```python
from build123d import *

# Parameters (mm, degrees)
SKETCH_1_R          = 18
LASHENA_DEPTH       = 30
CUT_EXTRUDEA_DEPTH  = 30
WWW_KYTOOL_CN_COUNT = 16
SKETCH_3_W          = 35.542909486
SKETCH_3_H          = 27
CUT_EXTRUDE_2_DEPTH = 30
SKETCH_4_R          = 1.5
CUT_EXTRUDE_3_DEPTH = 60
SKETCH_5_R          = 1.5
EXTRUDE_3_DEPTH     = 3
CUT_EXTRUDE_5_DEPTH = 3


with BuildPart() as part:
    # 草图1 → LaShenA (new body)
    with BuildSketch(Plane.XY):
        Circle(SKETCH_1_R)
    extrude(amount=LASHENA_DEPTH)

    # SketchA → Cut-ExtrudeA (cut)
    with BuildSketch(Plane.XY.offset(30)):
        with BuildLine():
            ThreePointArc((0.423212707, 13.493364703), (0, 13.5), (-0.423212707, 13.493364703))
            ThreePointArc((-0.423212707, 13.493364703), (-0.952770902, 13.685686791), (-1.20440395, 14.18977059))
            add(Edge.make_bspline(
                [(-1.20440395, 14.18977059), (-1.226562505, 14.455224305), (-1.213843633, 14.773889884), (-1.273675597, 15.110607864), (-1.299119688, 15.21139578), (-1.321432077, 15.29109757), (-1.349914152, 15.382250837), (-1.385146673, 15.484587535), (-1.427834192, 15.597770763), (-1.478623281, 15.721446817), (-1.538159915, 15.855229004), (-1.607069773, 15.998703507), (-1.685962928, 16.151428337), (-1.775430978, 16.312934487), (-1.876046532, 16.482726463), (-1.98836201, 16.660283053), (-2.112908684, 16.845058076), (-2.250195688, 17.036481179), (-2.400709063, 17.233958676), (-2.56491084, 17.43687441), (-2.743238138, 17.644590662), (-2.936102365, 17.856449073), (-3.14388814, 18.07177164), (-3.447378451, 18.368492697), (-3.689495989, 18.585006365), (-3.858042439, 18.727457792)],
                knots=[0.122308221, 0.122308221, 0.122308221, 0.122308221, 0.250610689, 0.276296194, 0.287604067, 0.300967916, 0.316387742, 0.333863545, 0.353395324, 0.37498308, 0.398626813, 0.424326522, 0.452082207, 0.48189387, 0.513761509, 0.547685125, 0.583664717, 0.621700286, 0.661791832, 0.703939355, 0.748142854, 0.79440233, 0.842717782, 0.893089212, 1, 1, 1, 1], degree=3))
            ThreePointArc((-3.858042439, 18.727457792), (0, 19.120726106), (3.858042439, 18.727457792))
            add(Edge.make_bspline(
                [(1.20440395, 14.18977059), (1.226562505, 14.455224305), (1.213843633, 14.773889884), (1.273675597, 15.110607864), (1.299119688, 15.21139578), (1.321432077, 15.29109757), (1.349914152, 15.382250837), (1.385146673, 15.484587535), (1.427834192, 15.597770763), (1.478623281, 15.721446817), (1.538159915, 15.855229004), (1.607069773, 15.998703507), (1.685962928, 16.151428337), (1.775430978, 16.312934487), (1.876046532, 16.482726463), (1.98836201, 16.660283053), (2.112908684, 16.845058076), (2.250195688, 17.036481179), (2.400709063, 17.233958676), (2.56491084, 17.43687441), (2.743238138, 17.644590662), (2.936102365, 17.856449073), (3.14388814, 18.07177164), (3.447378451, 18.368492697), (3.689495989, 18.585006365), (3.858042439, 18.727457792)],
                knots=[0.122308221, 0.122308221, 0.122308221, 0.122308221, 0.250610689, 0.276296194, 0.287604067, 0.300967916, 0.316387742, 0.333863545, 0.353395324, 0.37498308, 0.398626813, 0.424326522, 0.452082207, 0.48189387, 0.513761509, 0.547685125, 0.583664717, 0.621700286, 0.661791832, 0.703939355, 0.748142854, 0.79440233, 0.842717782, 0.893089212, 1, 1, 1, 1], degree=3))
            ThreePointArc((1.20440395, 14.18977059), (0.952770902, 13.685686791), (0.423212707, 13.493364703))
        make_face()
    cut_extrudea = extrude(amount=-CUT_EXTRUDEA_DEPTH, mode=Mode.SUBTRACT)

    # www.KYTool.cn: Cut-ExtrudeA ×16 about axis
    www_kytool_cn_axis = Axis((0, 0, -80.9), (0, 0, 1))
    for i in range(1, WWW_KYTOOL_CN_COUNT):
        add(cut_extrudea.rotate(www_kytool_cn_axis, i * 360 / WWW_KYTOOL_CN_COUNT), mode=Mode.SUBTRACT)

    # 草图3 → 切除-拉伸2 (cut, symmetric)
    with BuildSketch(Plane(origin=(0, 0, 0), x_dir=(1, 0, 0), z_dir=(0, 1, 0))):
        with Locations((0, -13.5)):
            Rectangle(SKETCH_3_W, SKETCH_3_H)
    extrude(amount=CUT_EXTRUDE_2_DEPTH, both=True, mode=Mode.SUBTRACT)

    # 草图4 → 切除-拉伸3 (cut)
    with BuildSketch(Plane.XY.offset(30)):
        Circle(SKETCH_4_R)
    extrude(amount=-CUT_EXTRUDE_3_DEPTH, mode=Mode.SUBTRACT)

    # 草图5 → 凸台-拉伸3 (add)
    with BuildSketch(Plane.XY.offset(30)):
        with BuildLine():
            Line((15.280220873, -61.835446614), (7.518552247, -73.648578352))
            ThreePointArc((7.518552247, -73.648578352), (6.801054577, -77.407548694), (8.951700529, -80.572889581))
            Line((8.951700529, -80.572889581), (9.765341245, -81.107481911))
            ThreePointArc((9.765341245, -81.107481911), (13.973775635, -81.709971806), (17.124630908, -78.855847572))
            Line((17.124630908, -78.855847572), (26.13082512, -57.293888764))
            ThreePointArc((26.13082512, -57.293888764), (26.903397768, -53.454512274), (26.142204066, -49.612863608))
            Line((26.142204066, -49.612863608), (9.545941546, -9.545941546))
            Line((9.545941546, -9.545941546), (0, -13.5))
            Line((0, -13.5), (16.161556687, -52.517449343))
            ThreePointArc((16.161556687, -52.517449343), (16.878328365, -57.285923538), (15.280220873, -61.835446614))
        make_face()
        with Locations((16.903408741, -40.017494037)):
            Circle(SKETCH_5_R, mode=Mode.SUBTRACT)
        with Locations((12.510922719, -76.928752156)):
            Circle(SKETCH_5_R, mode=Mode.SUBTRACT)
    extrude(amount=-EXTRUDE_3_DEPTH)

    # 草图8 → 切除-拉伸5 (cut)
    with BuildSketch(Plane.XY.offset(30)):
        with BuildLine():
            Line((-47.449101502, -4.18243968), (9.857223077, -40.017494037))
            ThreePointArc((9.857223077, -40.017494037), (14.412678985, -33.42621209), (22.188716957, -35.357638944))
            Line((22.188716957, -35.357638944), (66.6397739, 3.833166133))
            Line((66.6397739, 3.833166133), (-5.431022365, 32.995833694))
            Line((-5.431022365, 32.995833694), (-47.449101502, -4.18243968))
        make_face()
    extrude(amount=-CUT_EXTRUDE_5_DEPTH, mode=Mode.SUBTRACT)


solid = part.part
```
Model file for the job. Use its own axes, mm. A direction names the side the tool comes from. Give positions to 0.01 mm unless a question says otherwise; leave off trailing zeros. Write each loop counter-clockwise with the first axis right and the second up, starting at its lowest first coordinate (ties: lowest second). Pieces come first, ordered by that corner, then holes. Notation, with made-up numbers: (12, -21.75) - (70, -21.75) arc R36 ccw to (70, 12.25) - close; hole circle Ø8 at (88, -29.75). An arc over 180 degrees is marked (long way). One line per question, with ' | ' between items. Start each with the question number.
(1) Slice it at B-B on z = 29.05. Write the cut outline in (x, y), plus the area to 3 significant figures.
(2) Slice it at C-C on y = -64.5. Write the cut outline in (x, z), plus the area to 3 significant figures.
(3) Wall check: line 1 along Y through (x, z) = (13.5, 27.7); line 2 along Y through (x, z) = (10.5, 27.4); line 3 along X through (y, z) = (-41, 27.4). Give the ranges that are in metal, low to high. Write a range as from..to.
(4) Slice it at A-A on x = 11.5. Write the cut outline in (y, z).
(5) 3-axis set-ups, long thin cutter, end or side, ignore diameter. For faces 1 (the face through (13.317, -75.664, 28.521)), 2 (the face through (11.454, -67.659, 28.521)): which of +Z, -Z, +X, -X, +Y, -Y reach the whole face in a straight line?
(6) Slice it at D-D on x = 22.5. Write the cut outline in (y, z), plus the area to 3 significant figures.
(7) Pin check, flat tips, straight feed: P1, Ø1, axis at x = 21.5, z = 29, coming from the +Y side; P2, Ø2.5, axis at x = 16.9, y = -40.02, coming from the +Z side; P3, Ø3.5, axis at x = 12.51, y = -76.93, coming from the -Z side. Stop position of each tip, or through.
(8) Two-plate mould, pull along X, no slides. Class faces 3 (the face through (16.885, -57.218, 28.521)), 4 (the face through (21.565, -68.226, 28.521)), 5 (the face through (15.8, -39, 28.5)), 6 (the face through (13.91, -81.73, 28.52)): +X half, -X half, draft (parallel to the pull), parting line (faces both ways), or undercut.
Results below:
1) outline: (7.52, -73.65) arc R5 ccw to (8.95, -80.57) - (9.77, -81.11) arc R5 ccw to (17.12, -78.86) - (26.13, -57.29) arc R10 ccw to (26.14, -49.61) - (19.45, -33.45) arc R7.05 ccw to (10.15, -38.01) - (16.16, -52.52) arc R10 cw to (15.28, -61.84) - close; hole circle Ø3 at (12.51, -76.93); hole circle Ø3 at (16.9, -40.02) | area: 480 mm^2
2) outline: (13.53, 27) - (23.12, 27) - (23.12, 30) - (13.53, 30) - close | area: 28.8 mm^2
3) line 1: -81.83..-78.06, -75.8..-64.54, -46.09..-33.85 | line 2: -81.51..-69.11, -38.85..-37.08 | line 3: 11.39..15.77, 18.04..22.57
4) outline: (-81.83, 27) - (-78.04, 27) - (-78.04, 30) - (-81.83, 30) - close; (-75.82, 27) - (-67.59, 27) - (-67.59, 30) - (-75.82, 30) - close; (-41.26, 27) - (-35.5, 27) - (-35.5, 30) - (-41.26, 30) - close
5) face 1: +Z, -Z | face 2: +Z, -Z, -X
6) outline: (-65.99, 27) - (-40.82, 27) - (-40.82, 30) - (-65.99, 30) - close | area: 75.5 mm^2
7) P1: y = -37.2 | P2: through | P3: z = 27
8) face 3: -X half | face 4: +X half | face 5: undercut | face 6: parting line
